Can you work these out from the model? Positions are in its coordinate system, mm. Give positions to 0.01 mm unless a question says otherwise; leave off trailing zeros. Order: outer loops, then holes, each group sorted by start corner. A loop starts at its lowest first (then second) coordinate and runs counter-clockwise, first axis right, second up. Notation, with made-up numbers: (-1, 32) - (34, 32) arc R11 cw to (34, 40) - close; hole circle Ø1 at (68.25, 46). An arc over 180 degrees is marked (long way). Use one line per item in the form item = value. Start each with the question number.
1) Suppose I cut it at A-A, the plane y = -6.5. Write out the boundary of the cut face in (x, z) (3 decimals).
2) Please list where these lines run through material, in increasing order: probe 1 along X at (y, z) = (-2, 1.15) (3 decimals); probe 2 along X at (y, z) = (-15.5, 2.8); probe 3 along Y at (x, z) = (44.5, 1.4) (3 decimals).
3) Suppose I cut it at D-D, the plane x = -5. Write out the boundary of the cut face in (y, z) (3 decimals), and give its area (3 significant figures).
4) For pin 1 (1.6 mm diameter, centred on x = -7.5, z = 1, fed in from -Y); pin 2 (1 mm diameter, centred on x = 42.5, z = 2, fed in from +Y); pin 3 (5.5 mm diameter, centred on x = 40.576, y = 7.77, fed in from -Z), each with a flat end and sliding along its axis, tell me the tip position at first contact or that it passes through.
5) Suppose I cut it at B-B, the plane z = 2.55. Write out the boundary of the cut face in (x, y) (3 decimals), and give its area (3 significant figures).
6) Suppose I cut it at C-C, the plane x = -24. Write out the boundary of the cut face in (y, z) (3 decimals).
```python
from build123d import *

# Parameters (mm, degrees)
SKETCH1_W            = 6.266
SKETCH1_H            = 19.6
SKETCH1_R            = 1.675
SKETCH1_W_2          = 52.832
SKETCH1_H_2          = 5
BOSS_EXTRUDE2_DEPTH  = 3.175
SKETCH3_W            = 30
SKETCH3_H            = 29.6
BOSS_EXTRUDE3_DEPTH  = 3.175
SKETCH4_R            = 4.75
CUT_EXTRUDE1_DEPTH   = 10
BOSS_EXTRUDE14_DEPTH = 3.175
CUT_EXTRUDE8_DEPTH   = 10
BOSS_EXTRUDE15_DEPTH = 3.175
BOSS_EXTRUDE16_DEPTH = 3.175
BOSS_EXTRUDE17_DEPTH = 3.175
FILLET5_R            = 4
SKETCH27_W           = 3.175
SKETCH27_H           = 8
CUT_EXTRUDE9_DEPTH   = 10
SKETCH28_W           = 18
SKETCH28_H           = 3.175
BOSS_EXTRUDE18_DEPTH = 3.175
SKETCH29_W           = 53.813797415
SKETCH29_H           = 23.475817665
BOSS_EXTRUDE19_DEPTH = 3.175


with BuildPart() as part:
    # Sketch1 → Boss-Extrude2 (new body)
    # profile 1 of 4: a face of its own
    with BuildSketch(Plane.XY):
        with Locations((-23.283, 0)):
            Rectangle(SKETCH1_W, SKETCH1_H)
        with Locations((-23.95, -4.974)):
            Circle(SKETCH1_R, mode=Mode.SUBTRACT)
        with Locations((-23.95, 4.974)):
            Circle(SKETCH1_R, mode=Mode.SUBTRACT)
    # profile 2 of 4: a face of its own
    with BuildSketch(Plane.XY):
        with Locations((23.283, 0)):
            Rectangle(SKETCH1_W, SKETCH1_H)
        with Locations((23.95, -4.974)):
            Circle(SKETCH1_R, mode=Mode.SUBTRACT)
        with Locations((23.95, 4.974)):
            Circle(SKETCH1_R, mode=Mode.SUBTRACT)
    # profile 3 of 4: a face of its own
    with BuildSketch(Plane.XY):
        with Locations((0, 12.3)):
            Rectangle(SKETCH1_W_2, SKETCH1_H_2)
    # profile 4 of 4: a face of its own
    with BuildSketch(Plane.XY):
        with Locations((0, -12.3)):
            Rectangle(SKETCH1_W_2, SKETCH1_H_2)
    extrude(amount=BOSS_EXTRUDE2_DEPTH)

    # Sketch3 → Boss-Extrude3 (add)
    with BuildSketch(Plane.XY.offset(3.175)):
        with Locations((41.416, 0)):
            Rectangle(SKETCH3_W, SKETCH3_H)
    extrude(amount=-BOSS_EXTRUDE3_DEPTH)

    # Sketch4 → Cut-Extrude1 (cut)
    with BuildSketch(Plane(origin=(0, 0, 0), x_dir=(-1, 0, 0), z_dir=(0, 0, -1))):
        with Locations((-40.576, 7.77)):
            Circle(SKETCH4_R)
    extrude(amount=-CUT_EXTRUDE1_DEPTH, mode=Mode.SUBTRACT)

    # Sketch22 → Boss-Extrude14 (add)
    with BuildSketch(Plane(origin=(0, 0, 0), x_dir=(-1, 0, 0), z_dir=(0, 0, -1))):
        with BuildLine():
            ThreePointArc((-34.680262133, 14.8), (-40.576, 16.945), (-46.471737867, 14.8))
            Line((-46.471737867, 14.8), (-34.680262133, 14.8))
        make_face()
    extrude(amount=-BOSS_EXTRUDE14_DEPTH)

    # Sketch23 → Cut-Extrude8 (cut)
    with BuildSketch(Plane(origin=(0, 0, 0), x_dir=(-1, 0, 0), z_dir=(0, 0, -1))):
        with BuildLine():
            Line((-49.751, -14.8), (-49.751, 7.77))
            ThreePointArc((-49.751, 7.77), (-48.890866804, 11.648609936), (-46.471737867, 14.8))
            Line((-46.471737867, 14.8), (-56.416, 14.8))
            Line((-56.416, 14.8), (-56.416, -14.8))
            Line((-56.416, -14.8), (-49.751, -14.8))
        make_face()
    extrude(amount=-CUT_EXTRUDE8_DEPTH, mode=Mode.SUBTRACT)

    # Sketch24 → Boss-Extrude15 (add)
    with BuildSketch(Plane(origin=(0, 0, 0), x_dir=(-1, 0, 0), z_dir=(0, 0, -1))):
        Polygon((30.625, 14.8), (26.416, 14.8), (26.416, -14.8), (27.751006616, -14.8), (30.625, -14.8), align=None)
    extrude(amount=-BOSS_EXTRUDE15_DEPTH)

    # Sketch25 → Boss-Extrude16 (add)
    with BuildSketch(Plane(origin=(0, 0, 0), x_dir=(-1, 0, 0), z_dir=(0, 0, -1))):
        Polygon((30.625, 14.8), (30.625, 9.8), (33.8, 9.8), (33.8, 1.8), (30.625, 1.8), (30.625, -1.8), (33.8, -1.8), (33.8, -9.8), (30.625, -9.8), (30.625, -14.8), (31.879074074, -14.8), (38.8, -14.8), (38.8, 14.8), align=None)
    extrude(amount=-BOSS_EXTRUDE16_DEPTH)

    # Sketch26 → Boss-Extrude17 (add)
    with BuildSketch(Plane(origin=(0, 0, 0), x_dir=(-1, 0, 0), z_dir=(0, 0, -1))):
        with BuildLine():
            ThreePointArc((-40.225848077, 16.938316019), (-37.275108655, 16.330650754), (-34.680262133, 14.8))
            Line((-34.680262133, 14.8), (38.8, 14.8))
            ThreePointArc((38.8, 14.8), (-0.708684686, 16.025831975), (-40.225848077, 16.938316019))
        make_face()
    extrude(amount=-BOSS_EXTRUDE17_DEPTH)

    # Fillet5
    fillet5_edges = [part.edges().sort_by_distance(p)[0] for p in [
        (-38.8, 14.8, 1.5875),
    ]]
    fillet(fillet5_edges, radius=FILLET5_R)

    # Sketch27 → Cut-Extrude9 (cut)
    with BuildSketch(Plane(origin=(0, 0, 0), x_dir=(-1, 0, 0), z_dir=(0, 0, -1))):
        with Locations((-43.1635, -5.8)):
            Rectangle(SKETCH27_W, SKETCH27_H)
    extrude(amount=-CUT_EXTRUDE9_DEPTH, mode=Mode.SUBTRACT)

    # Sketch28 → Boss-Extrude18 (add)
    with BuildSketch(Plane(origin=(0, 0, 0), x_dir=(-1, 0, 0), z_dir=(0, 0, -1))):
        with Locations((-40.751, -16.3875)):
            Rectangle(SKETCH28_W, SKETCH28_H)
        with Locations((-6.85, -16.3875)):
            Rectangle(SKETCH28_W, SKETCH28_H)
        with Locations((29.8, -16.3875)):
            Rectangle(SKETCH28_W, SKETCH28_H)
    extrude(amount=-BOSS_EXTRUDE18_DEPTH)

    # Sketch29 → Boss-Extrude19 (add)
    with BuildSketch(Plane(origin=(0, 0, 0), x_dir=(-1, 0, 0), z_dir=(0, 0, -1))):
        with Locations((0.393454416, 0.74908249)):
            Rectangle(SKETCH29_W, SKETCH29_H)
    extrude(amount=-BOSS_EXTRUDE19_DEPTH)


solid = part.part
```
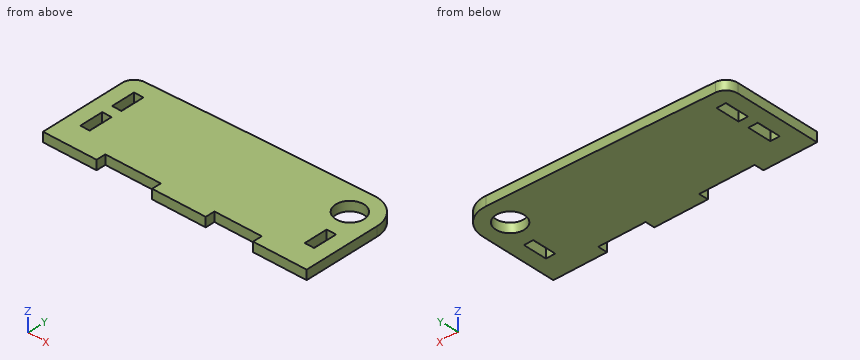
Result sheet:
q1.outline = (-38.8, 0) - (-33.8, 0) - (-33.8, 3.175) - (-38.8, 3.175) - close; (-30.625, 0) - (41.576, 0) - (41.576, 3.175) - (-30.625, 3.175) - close; (44.751, 0) - (49.751, 0) - (49.751, 3.175) - (44.751, 3.175) - close
q2.probe_1 = -38.8 to -33.8, -30.625 to 41.576, 44.751 to 49.751
q2.probe_2 = -38.8 to -20.8, -2.15 to 15.85, 31.75 to 49.75
q2.probe_3 = -17.975 to -9.8, -1.8 to 5.093, 10.447 to 16.064
q3.outline = (-14.8, 0) - (15.868, 0) - (15.868, 3.175) - (-14.8, 3.175) - close
q3.area = 97.4 mm²
q4.pin_1 = -14.8
q4.pin_2 = 16.83
q4.pin_3 = through
q5.outline = (-38.8, -17.975) - (-20.8, -17.975) - (-20.8, -14.8) - (-2.15, -14.8) - (-2.15, -17.975) - (15.85, -17.975) - (15.85, -14.8) - (31.751, -14.8) - (31.751, -17.975) - (49.751, -17.975) - (49.751, 7.77) arc R9.175 ccw to (40.226, 16.938) arc R4984.45 ccw to (-34.937, 14.934) arc R4 ccw to (-38.8, 10.936) - close; hole (-33.8, -9.8) - (-30.625, -9.8) - (-30.625, -1.8) - (-33.8, -1.8) - close; hole (-33.8, 1.8) - (-30.625, 1.8) - (-30.625, 9.8) - (-33.8, 9.8) - close; hole circle Ø9.5 at (40.576, 7.77); hole (41.576, -9.8) - (44.751, -9.8) - (44.751, -1.8) - (41.576, -1.8) - close
q5.area = 2,740 mm²
q6.outline = (-17.975, 0) - (15.296, 0) - (15.296, 3.175) - (-17.975, 3.175) - close
